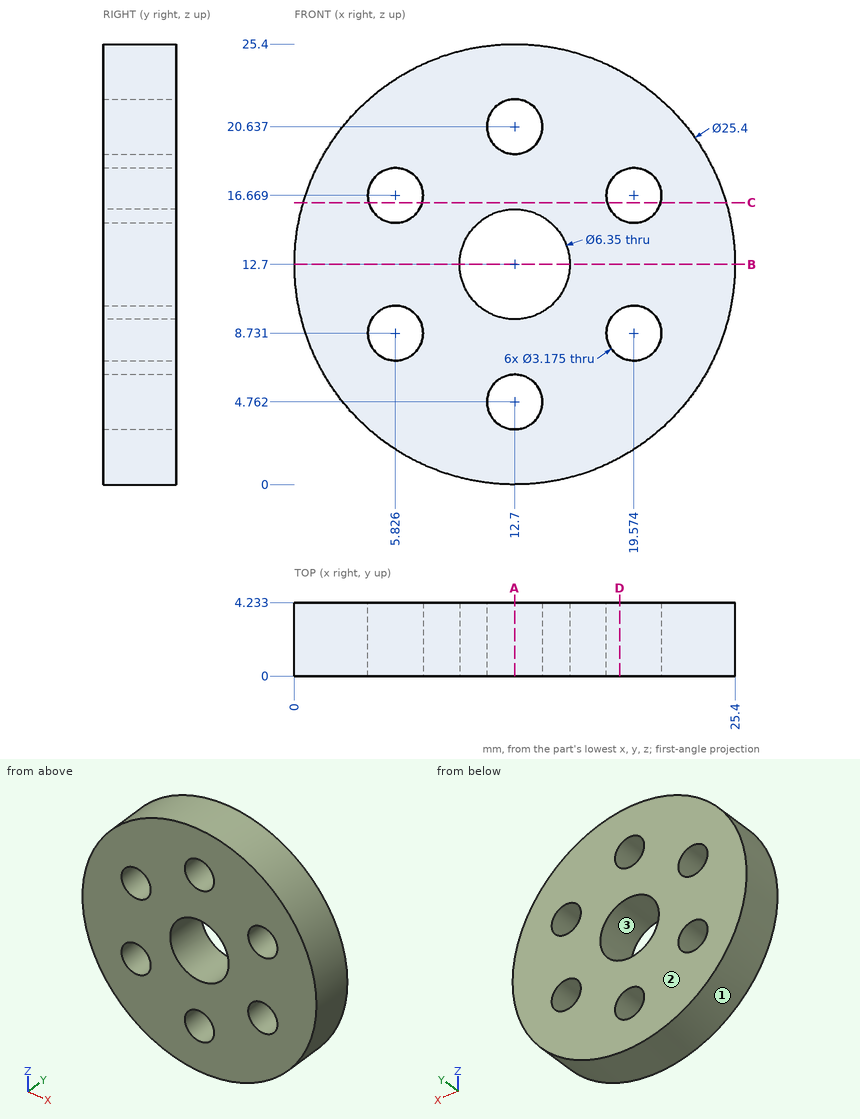
Source: three-view drawing plus pictorial views. Frame: mm from the lowest corner of the part. Round coordinates to 2 decimals unless told otherwise and drop trailing zeros. Loops run counter-clockwise (first coordinate to the right, second up) from the corner with the lowest first, then second, coordinate; pieces in that order, holes last.
Q1. Pin query (flat end, axial travel): P1, Ø1.5, axis at x = 11.5, y = 3.5, coming from the -Z side; P2, Ø4, axis at x = 12.7, z = 12.7, coming from the -Y side; P3, Ø1.5, axis at x = 4, y = 0.5, coming from the -Z side (1 decimal); P4, Ø2, axis at x = 17.5, y = 3.5, coming from the -Z side. Return the tip coordinate at first contact, or that it passes through.
Q2. Pull-direction query (Z, two-part tool) for the marked faces 1, 2 and 3; classes: released by +Z, released by -Z, zero draft, split by the parting line, or undercut.
Q3. Section C-C on z = 16.25. Return loops of the section in (x, y) (1 decimal).
Q4. Section B-B on z = 12.7. Return loops of the section in (x, y) (1 decimal).
Q5. Material intervals for L1, parallel to Z at x = 12, y = 1.55 (1 decimal); L2, parallel to X at y = 2.7, z = 9.25 (1 decimal); L3, parallel to X at y = 1.15, z = 15.25 (1 decimal), sorted ascending.
Q6. Section D-D on x = 18.75. Return loops of the section in (y, z) (1 decimal).
Q7. Section A-A on x = 12.7. State how many separate pieces and enclosed holes the cut face has.
Evaluation:
1. P1: stops at z = 0.01
1. P2: passes through
1. P3: stops at z = 2.8
1. P4: stops at z = 0.58
2. face 1: split by the parting line
2. face 2: zero draft
2. face 3: undercut
3. outline: (0.5, 0) - (4.3, 0) - (4.3, 4.2) - (0.5, 4.2) - close; (7.4, 0) - (18, 0) - (18, 4.2) - (7.4, 4.2) - close; (21.1, 0) - (24.9, 0) - (24.9, 4.2) - (21.1, 4.2) - close
4. outline: (0, 0) - (9.5, 0) - (9.5, 4.2) - (0, 4.2) - close; (15.9, 0) - (25.4, 0) - (25.4, 4.2) - (15.9, 4.2) - close
5. L1: z = 0 to 3.3, 6.2 to 9.6, 15.8 to 19.2, 22.1 to 25.4
5. L2: x = 0.5 to 4.3, 7.3 to 18.1, 21.1 to 24.9
5. L3: x = 0.3 to 5.1, 6.5 to 10.8, 14.6 to 18.9, 20.3 to 25.1
6. outline: (0, 1.5) - (4.2, 1.5) - (4.2, 7.4) - (0, 7.4) - close; (0, 10.1) - (4.2, 10.1) - (4.2, 15.3) - (0, 15.3) - close; (0, 18) - (4.2, 18) - (4.2, 23.9) - (0, 23.9) - close
7. separate pieces: 4
7. enclosed holes: 0
